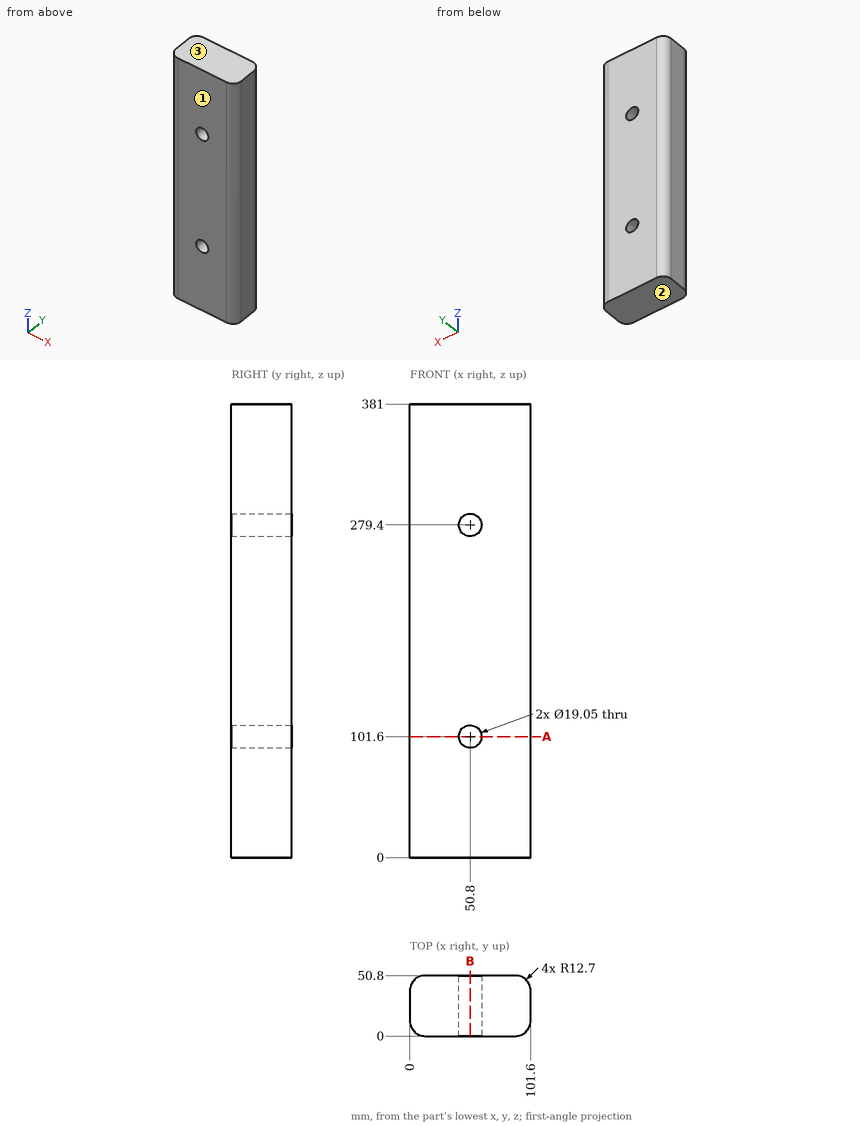
Source: three-view drawing plus pictorial views. Frame: mm from the lowest corner of the part. Round coordinates to 2 decimals unless told otherwise and drop trailing zeros. Loops run counter-clockwise (first coordinate to the right, second up) from the corner with the lowest first, then second, coordinate; pieces in that order, holes last.
Q1. Pull-direction query (Z, two-part tool) for the marked faces 1, 2 and 3; classes: released by +Z, released by -Z, zero draft, split by the parting line, or undercut.
Q2. Section A-A on z = 101.6. Return loops of the section in (x, y) (3 decimals).
Q3. Material intervals for L1, parallel to Z at x = 50, y = 27; L2, parallel to X at y = 19, z = 279.4 (3 decimals); L3, parallel to Z at x = 56.5, y = 6.5, sorted ascending.
Q4. Pin query (flat end, axial travel): P1, Ø17, axis at x = 50.8, z = 101.6, coming from the -Y side. Return the tip coordinate at first contact, or that it passes through.
Q5. Section B-B on x = 50.8. Return loops of the section in (y, z) (3 decimals).
Evaluation:
1. face 1: zero draft
1. face 2: released by -Z
1. face 3: released by +Z
2. outline: (0, 12.7) arc R12.7 ccw to (12.7, 0) - (41.275, 0) - (41.275, 50.8) - (12.7, 50.8) arc R12.7 ccw to (0, 38.1) - close; (60.325, 0) - (88.9, 0) arc R12.7 ccw to (101.6, 12.7) - (101.6, 38.1) arc R12.7 ccw to (88.9, 50.8) - (60.325, 50.8) - close
3. L1: z = 0 to 92.11, 111.09 to 269.91, 288.89 to 381
3. L2: x = 0 to 41.275, 60.325 to 101.6
3. L3: z = 0 to 93.97, 109.23 to 271.77, 287.03 to 381
4. P1: passes through
5. outline: (0, 0) - (50.8, 0) - (50.8, 92.075) - (0, 92.075) - close; (0, 111.125) - (50.8, 111.125) - (50.8, 269.875) - (0, 269.875) - close; (0, 288.925) - (50.8, 288.925) - (50.8, 381) - (0, 381) - close
